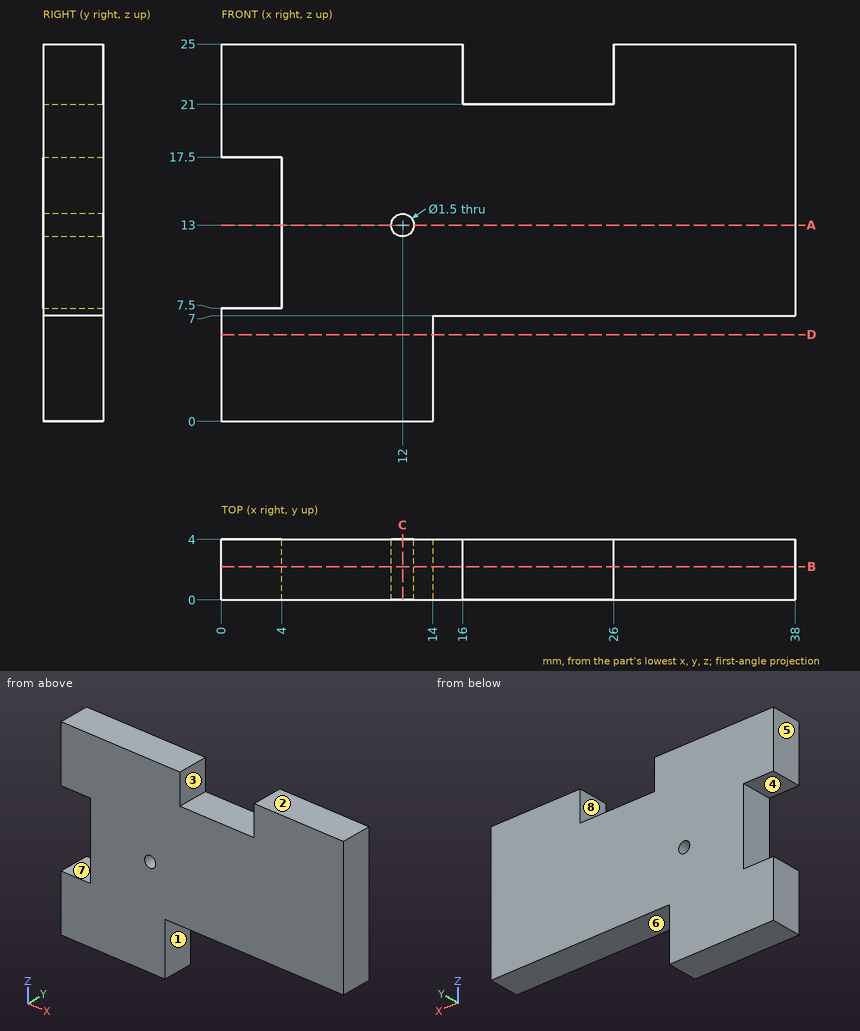
Source: three-view drawing plus pictorial views. Frame: mm from the lowest corner of the part. A direction names the side the tool comes from. Give positions to 0.01 mm unless a question says otherwise; leave off trailing zeros. Order: outer loops, then holes, each group sorted by start corner. A loop starts at its lowest first (then second) coordinate and runs counter-clockwise, first axis right, second up. Notation, with made-up numbers: M 48,-9.5 L 104,-9.5 A28 cw 104,28.5 Z; hole C 31,-30.5 d9. An arc over 180 degrees is marked long. Return JSON: item names as keys, results as strings.
Item 1: First-contact query: P1, Ø1.2, axis at x = 22, y = 2, coming from the -Z side; P2, Ø1.2, axis at x = 22, y = 2, coming from the +Z side; P3, Ø2, axis at y = 1, z = 3.5, coming from the +X side; P4, Ø2, axis at y = 2, z = 22.5, coming from the -X side. Flat tips, straight axial feed; report the tip coordinate or a pass-through.
Solutions:
{"P1": "z = 7", "P2": "z = 21", "P3": "x = 14", "P4": "x = 0"}
Item 2: Access query for the marked faces 1, 2, 3, 4 and 5. Directions: +Z, -Z, +X, -X, +Y, -Y. A direction counts if a zero-diameter tool reaches every point of the face in a straight line with its end or side. Return the directions, or none.
Solutions:
{"face 1": "-Z, +X, +Y, -Y", "face 2": "+Z, +X, -X, +Y, -Y", "face 3": "+Z, +Y, -Y", "face 4": "-X, +Y, -Y", "face 5": "+Z, -Z, -X, +Y, -Y"}
Item 3: Cut plane B-B (y = 2.2). Return loops of the section in (x, z).
Solutions:
{"outline": "M 0,0 L 14,0 L 14,7 L 38,7 L 38,25 L 26,25 L 26,21 L 16,21 L 16,25 L 0,25 L 0,17.5 L 4,17.5 L 4,7.5 L 0,7.5 Z; hole C 12,13 d1.5"}
Item 4: Cut plane C-C (x = 12). Return loops of the section in (y, z).
Solutions:
{"outline": "M 0,0 L 4,0 L 4,12.25 L 0,12.25 Z; M 0,13.75 L 4,13.75 L 4,25 L 0,25 Z"}
Item 5: Ray query, probe 1 along X at (y, z) = (2.9, 13); probe 2 along Z at (x, y) = (2.5, 3.6); probe 3 along Z at (x, y) = (36, 0.75). Return the intervals inside material, ascending.
Solutions:
{"probe 1": "4 to 11.25, 12.75 to 38", "probe 2": "0 to 7.5, 17.5 to 25", "probe 3": "7 to 25"}
Item 6: Cut plane A-A (z = 13). Return loops of the section in (x, y), then the cut area to 3 significant figures.
Solutions:
{"outline": "M 4,0 L 11.25,0 L 11.25,4 L 4,4 Z; M 12.75,0 L 38,0 L 38,4 L 12.75,4 Z", "area": "130 mm^2"}
Item 7: Cut plane D-D (z = 5.75). Return loops of the section in (x, y).
Solutions:
{"outline": "M 0,0 L 14,0 L 14,4 L 0,4 Z"}
Item 8: Pull-direction query (Z, two-part tool) for the marked faces 6, 7 and 8; classes: +Z half, -Z half, draft (parallel to the pull), parting line (faces both ways), or undercut.
Solutions:
{"face 6": "-Z half", "face 7": "undercut", "face 8": "draft"}
